Geometry check sheet. Reference: the model listing, model coordinates, mm. A direction names the side the tool comes from. Round coordinates to 2 decimals unless told otherwise and drop trailing zeros. Write each loop counter-clockwise with the first axis right and the second up, starting at its lowest first coordinate (ties: lowest second). Pieces come first, ordered by that corner, then holes.
from build123d import *

# Parameters (mm, degrees)
F1_DEPTH = 120
F3_D     = 10
F5_D     = 6
F6_R     = 5


with BuildPart() as f1:
    # F0 (on Top) → F1 (new body)
    with BuildSketch(Plane.XY):
        Polygon((30, 0), (0, 0), (0, -2), (32, -2), (32, 24), (0, 24), (0, 22), (30, 22), align=None)
    extrude(amount=F1_DEPTH)

    # F3 (through all)
    with Locations(Plane.XZ.offset(2)):
        with Locations((10, 110), (10, 10)):
            Hole(F3_D / 2)

    # F5 (through all)
    with Locations(Plane.YZ.offset(32)):
        with Locations((11, 60)):
            Hole(F5_D / 2)

    # F6
    f6_edges = [f1.edges().sort_by_distance(p)[0] for p in [
        (0, -1, 120),
        (0, 23, 120),
        (0, 23, 0),
        (0, -1, 0),
    ]]
    fillet(f6_edges, radius=F6_R)


solid = f1.part
1. Section check B-B (y = 11). Record the cut outline in (x, z).
2. Section check D-D (x = 10). Record the cut outline in (y, z).
3. Section check C-C (x = 28). Record the cut outline in (y, z).
4. Section check A-A (z = 110). Record the cut outline in (x, y).
5. Release check for a two-part mould opening along Z. For faces 1 (the face through (5.23, 23.01, 111.5)), 2 (the face through (32, 8, 59)), 3 (the face through (2, 23, 1)), 4 (the face through (2, 23, 119)) record: +Z half, -Z half, draft (parallel to the pull), parting line (faces both ways), or undercut.
6. Scan lines: line 1 along Z through (x, y) = (10, 23.2); line 2 along Y through (x, z) = (27.5, 101.5); line 3 along Z through (x, y) = (31.25, 11). Record each from-to range of solid material in increasing order.
7. Access from +Z, -Z, +X, -X, +Y, -Y to the whole of each face (thin tool, end or side, straight path). Record for faces 5 (the face through (15, 22, 59)), 6 (the face through (0, 23, 59)).
8. Depth check by flat-ended pin: pin 1 Ø1 at (y, z) = (16.5, 103.5) entering from -X. Enter the tip coordinate at first touch or a pass-through.
Results below:
1. outline: (30, 0) - (32, 0) - (32, 57) - (30, 57) - close; (30, 63) - (32, 63) - (32, 120) - (30, 120) - close
2. outline: (-2, 0) - (0, 0) - (0, 5) - (-2, 5) - close; (-2, 15) - (0, 15) - (0, 105) - (-2, 105) - close; (-2, 115) - (0, 115) - (0, 120) - (-2, 120) - close; (22, 0) - (24, 0) - (24, 5) - (22, 5) - close; (22, 15) - (24, 15) - (24, 105) - (22, 105) - close; (22, 115) - (24, 115) - (24, 120) - (22, 120) - close
3. outline: (-2, 0) - (0, 0) - (0, 120) - (-2, 120) - close; (22, 0) - (24, 0) - (24, 120) - (22, 120) - close
4. outline: (0, -2) - (5, -2) - (5, 0) - (0, 0) - close; (0, 22) - (5, 22) - (5, 24) - (0, 24) - close; (15, -2) - (32, -2) - (32, 24) - (15, 24) - (15, 22) - (30, 22) - (30, 0) - (15, 0) - close
5. face 1: undercut
5. face 2: draft
5. face 3: -Z half
5. face 4: +Z half
6. line 1: z = 0 to 5, 15 to 105, 115 to 120
6. line 2: y = -2 to 0, 22 to 24
6. line 3: z = 0 to 57, 63 to 120
7. face 5: +Z, -Z, -X
7. face 6: +Z, -Z, -X, +Y, -Y
8. pin 1: stops at x = 30
